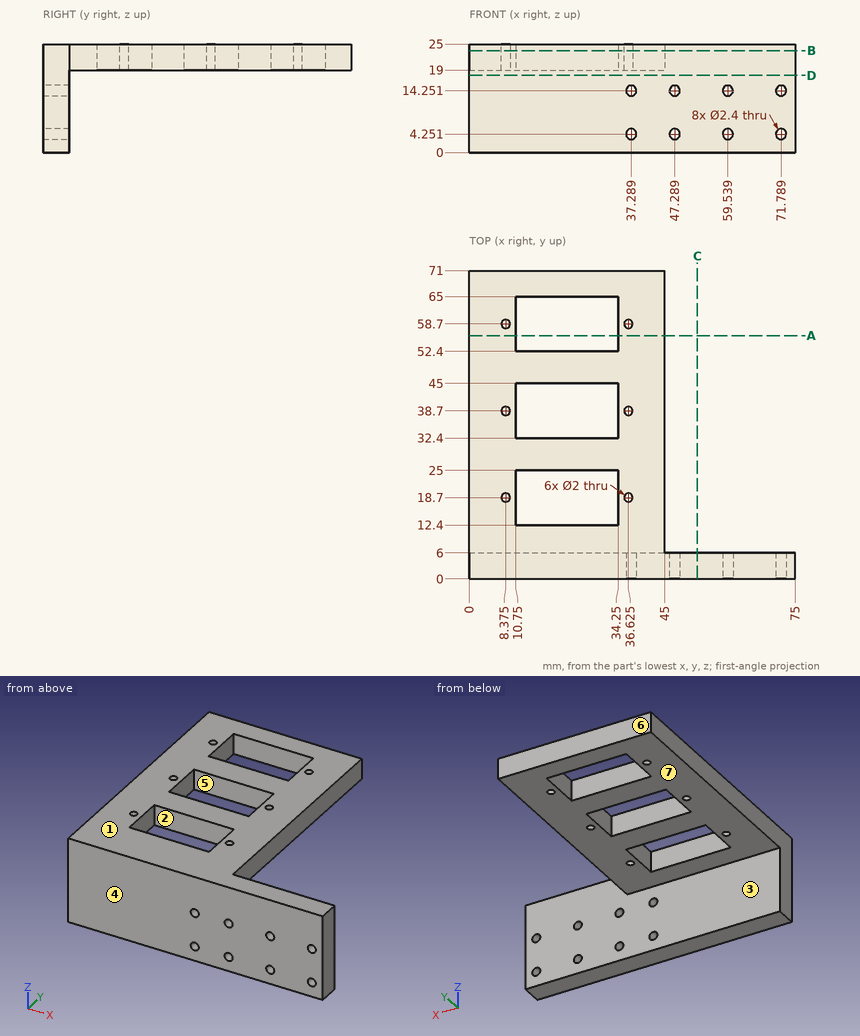
Geometry check sheet. Reference: drawing and pictorial views, mm from the part's lowest x, y, z. A direction names the side the tool comes from. Round coordinates to 2 decimals unless told otherwise and drop trailing zeros. Loops run counter-clockwise (first coordinate to the right, second up) from the corner with the lowest first, then second, coordinate; pieces in that order, holes last. Notation, with made-up numbers: (-33, 70) -> (24, 70) arc R17 ccw to (24, 93) -> close; hole circle Ø8 at (19.5, 87). An arc over 180 degrees is marked (long way). Answer as a JSON object with one key per item and string values. Group by question number.
Item 1: Depth check by flat-ended pin: pin 1 Ø2 at (x, z) = (53, 13.5) entering from -Y; pin 2 Ø4 at (x, z) = (13, 16.5) entering from +Y; pin 3 Ø5 at (y, z) = (20.5, 23) entering from +X; pin 4 Ø5 at (x, y) = (28, 12) entering from -Z. Enter the tip coordinate at first touch or a pass-through.
Item 2: Set-up check for the marked faces 5, 6 and 7: record each of +Z, -Z, +X, -X, +Y, -Y from which the full face is reachable in a straight line by a thin tool's end or side.
Item 3: Thickness scan on line 1 along X through (y, z) = (20, 23.25); line 2 along Z through (x, y) = (58.5, 3.5); line 3 along Y through (x, z) = (19.5, 14). Record the ranges inside material, lowest first.
Item 4: Cross-section at D-D, the plane z = 17.75. Record the cut outline in (x, y).
Item 5: Release check for a two-part mould opening along Y. For the marked faces 1, 2, 3 and 4 record: pulls with the +Y half, pulls with the -Y half, needs draft (parallel to the pull), parting line crosses it, or undercut.
Item 6: Cross-section at C-C, the plane x = 52.5. Record the cut outline in (y, z), plus the area to 3 significant figures.
Item 7: Cross-section at A-A, the plane y = 56. Record the cut outline in (x, z), plus the area to 3 significant figures.
Item 8: Cross-section at B-B, the plane z = 23.5. Count the separate pieces of the cut face and the enclosed holes in it, plus the area to 3 significant figures.
Determined:
{
 "1": {"pin 1": "stops at y = 0", "pin 2": "stops at y = 6", "pin 3": "stops at x = 45", "pin 4": "stops at z = 19"},
 "2": {"face 5": "+Z, -Z", "face 6": "+Z, -Z, +X, -X, +Y", "face 7": "-Z, +X, -X, +Y"},
 "3": {"line 1": "x = 0 to 10.75, 34.25 to 45", "line 2": "z = 0 to 3.65, 4.85 to 13.65, 14.85 to 25", "line 3": "y = 0 to 6"},
 "4": {"outline": "(0, 0) -> (75, 0) -> (75, 6) -> (0, 6) -> close"},
 "5": {"face 1": "needs draft", "face 2": "undercut", "face 3": "pulls with the +Y half", "face 4": "pulls with the -Y half"},
 "6": {"outline": "(0, 0) -> (6, 0) -> (6, 25) -> (0, 25) -> close", "area": "150 mm²"},
 "7": {"outline": "(0, 19) -> (10.75, 19) -> (10.75, 25) -> (0, 25) -> close; (34.25, 19) -> (45, 19) -> (45, 25) -> (34.25, 25) -> close", "area": "129 mm²"},
 "8": {"separate pieces": "1", "enclosed holes": "9", "area": "2,470 mm²"}
}
